Design review of the part built by this model. Coordinates are the model's own, in mm. Face numbers are marked on the shaded views. A direction names the side the tool comes from. Give positions to 0.01 mm unless a question says otherwise; leave off trailing zeros. Loops run counter-clockwise (first coordinate to the right, second up) from the corner with the lowest first, then second, coordinate; pieces in that order, holes last. Notation, with made-up numbers: (-18, 12) -> (8, 12) arc R11 cw to (8, 18) -> close; hole circle Ø4 at (13.25, 39.25). An arc over 180 degrees is marked (long way). Use a Markdown table: item, result. Add a question column.
1. Add section C-C (y = 15.5). State the section outline as (x, z) points.
2. To check wall thickness, follow line 1 (Y direction, x = 6, z = 19.75); line 2 (X direction, y = 8, z = 7.5); line 3 (X direction, y = 17, z = 27). State the ranges of each line that lie inside material, in increasing order.
3. Add section D-D (y = 27.5). State the section outline as (x, z) points.
4. Add section A-A (z = 12). State the section outline as (x, y) points.
5. For the marked faces 5 and 6, list the 3-axis set-ups (+Z, -Z, +X, -X, +Y, -Y) from which the entire face can be reached by the end or side of a thin tool; tool diameter is ignored.
6. For pin 1 Ø12 at (x, y) = (27.5, 25.5) entering from +Z; pin 2 Ø1.6 at (x, y) = (6.5, 27) entering from +Z; pin 3 Ø1.6 at (x, y) = (84, 4.5) entering from +Z; pin 4 Ø4.5 at (x, y) = (13, 16.5) entering from +Z, all flat-tipped, find the tip position at first contact; note any pin that passes through.
7. Draft analysis for pull direction Y (two halves, no side actions). For the marked faces 1, 2, 3 and 4, state which applies: pulls with the +Y half, pulls with the -Y half, needs draft (parallel to the pull), parting line crosses it, or undercut.
8. Add section B-B (x = 84). State the section outline as (y, z) points.
```python
from build123d import *

# Parameters (mm, degrees)
BOX_W           = 90
BOX_H           = 32
BOX_DEPTH       = 35
SKETCH_W        = 82
SKETCH_H        = 27
POCKET_DEPTH    = 30
SKETCH001_W     = 15
SKETCH001_H     = 27
PAD_DEPTH       = 20
SKETCH002_W     = 4
SKETCH002_H     = 4
PAD001_DEPTH    = 4
SKETCH003_W     = 2
SKETCH003_H     = 5
POCKET001_DEPTH = 6
SKETCH004_W     = 4.5
SKETCH004_H     = 2
POCKET002_DEPTH = 13
SKETCH005_W     = 5.5
SKETCH005_H     = 4.5
POCKET003_DEPTH = 2.5
FILLET_R        = 1
SKETCH006_R     = 1
POCKET004_DEPTH = 12
FILLET001_R     = 2


with BuildPart() as part:
    # Box → Box (new body)
    with BuildSketch(Plane.XY):
        with Locations((45, 16)):
            Rectangle(BOX_W, BOX_H)
    extrude(amount=BOX_DEPTH)

    # Sketch (on Face6 of BaseFeature) → Pocket (cut)
    with BuildSketch(Plane.XY.offset(35)):
        with Locations((45, 16)):
            Rectangle(SKETCH_W, SKETCH_H)
    extrude(amount=-POCKET_DEPTH, mode=Mode.SUBTRACT)

    # Sketch001 (on Face11 of Pocket) → Pad (join)
    with BuildSketch(Plane.XY.offset(5)):
        with Locations((11.5, 16)):
            Rectangle(SKETCH001_W, SKETCH001_H)
        with Locations((78.5, 16)):
            Rectangle(SKETCH001_W, SKETCH001_H)
    extrude(amount=PAD_DEPTH)

    # Sketch002 (on Face11 of Pad) → Pad001 (join)
    with BuildSketch(Plane.XY.offset(25)):
        with Locations((6, 27.5)):
            Rectangle(SKETCH002_W, SKETCH002_H)
        with Locations((6, 4.5)):
            Rectangle(SKETCH002_W, SKETCH002_H)
        with Locations((84, 27.5)):
            Rectangle(SKETCH002_W, SKETCH002_H)
        with Locations((84, 4.5)):
            Rectangle(SKETCH002_W, SKETCH002_H)
    extrude(amount=PAD001_DEPTH)

    # Sketch003 (on Face20 of Pad001) → Pocket001 (cut)
    with BuildSketch(Plane.XY.offset(25)):
        with Locations((76.5, 16)):
            Rectangle(SKETCH003_W, SKETCH003_H)
    extrude(amount=-POCKET001_DEPTH, mode=Mode.SUBTRACT)

    # Sketch004 (on Face6 of Pocket001) → Pocket002 (cut)
    with BuildSketch(Plane.YZ.offset(90)):
        with Locations((16, 20)):
            Rectangle(SKETCH004_W, SKETCH004_H)
    extrude(amount=-POCKET002_DEPTH, mode=Mode.SUBTRACT)

    # Sketch005 (on Face6 of Pocket002) → Pocket003 (cut)
    with BuildSketch(Plane.YZ.offset(90)):
        with Locations((16, 20)):
            Rectangle(SKETCH005_W, SKETCH005_H)
    extrude(amount=-POCKET003_DEPTH, mode=Mode.SUBTRACT)

    # Fillet
    fillet_edges = [part.edges().sort_by_distance(p)[0] for p in [
        (88.75, 13.25, 22.25),
        (88.75, 18.75, 22.25),
        (88.75, 13.25, 17.75),
        (88.75, 18.75, 17.75),
    ]]
    fillet(fillet_edges, radius=FILLET_R)

    # Sketch006 (on Face38 of Fillet) → Pocket004 (cut)
    with BuildSketch(Plane.XY.offset(29)):
        with Locations((84, 27.5)):
            Circle(SKETCH006_R)
        with Locations((84, 4.5)):
            Circle(SKETCH006_R)
        with Locations((6, 27.5)):
            Circle(SKETCH006_R)
        with Locations((6, 4.5)):
            Circle(SKETCH006_R)
    extrude(amount=-POCKET004_DEPTH, mode=Mode.SUBTRACT)

    # Fillet001
    fillet001_edges = [part.edges().sort_by_distance(p)[0] for p in [
        (0, 0, 17.5),
        (90, 0, 17.5),
        (90, 32, 17.5),
        (0, 32, 17.5),
    ]]
    fillet(fillet001_edges, radius=FILLET001_R)


solid = part.part
```
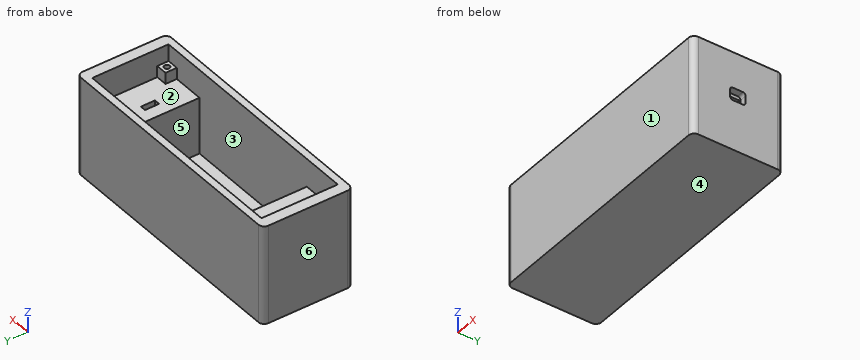
Taken from the geometry:
| question | item | result |
|---|---|---|
| 1 | outline | (0, 0) -> (90, 0) -> (90, 17.75) -> (87.5, 17.75) -> (87.5, 19) -> (75.5, 19) -> (75.5, 25) -> (71, 25) -> (71, 5) -> (19, 5) -> (19, 25) -> (4, 25) -> (4, 35) -> (0, 35) -> close; (77.5, 21) -> (87.5, 21) -> (87.5, 22.25) -> (90, 22.25) -> (90, 35) -> (86, 35) -> (86, 25) -> (77.5, 25) -> close |
| 2 | line 1 | y = 0 to 3.5, 5.5 to 26.5, 28.5 to 32 |
| 2 | line 2 | x = 0 to 19, 71 to 90 |
| 2 | line 3 | x = 0 to 4, 86 to 90 |
| 3 | outline | (0, 0) -> (90, 0) -> (90, 35) -> (86, 35) -> (86, 29) -> (85, 29) -> (85, 17) -> (83, 17) -> (83, 29) -> (82, 29) -> (82, 25) -> (71, 25) -> (71, 5) -> (19, 5) -> (19, 25) -> (8, 25) -> (8, 29) -> (7, 29) -> (7, 17) -> (5, 17) -> (5, 29) -> (4, 29) -> (4, 35) -> (0, 35) -> close |
| 4 | outline | (0, 2) arc R2 ccw to (2, 0) -> (88, 0) arc R2 ccw to (90, 2) -> (90, 30) arc R2 ccw to (88, 32) -> (2, 32) arc R2 ccw to (0, 30) -> close; hole (19, 2.5) -> (71, 2.5) -> (71, 29.5) -> (19, 29.5) -> close |
| 5 | face 5 | +Z |
| 5 | face 6 | +Z, -Z, -X, +Y, -Y |
| 6 | pin 1 | stops at z = 35 |
| 6 | pin 2 | stops at z = 29 |
| 6 | pin 3 | stops at z = 17 |
| 6 | pin 4 | stops at z = 25 |
| 7 | face 1 | pulls with the -Y half |
| 7 | face 2 | undercut |
| 7 | face 3 | undercut |
| 7 | face 4 | needs draft |
| 8 | outline | (0, 0) -> (32, 0) -> (32, 35) -> (29.5, 35) -> (29.5, 29) -> (28.5, 29) -> (28.5, 17) -> (26.5, 17) -> (26.5, 29) -> (25.5, 29) -> (25.5, 25) -> (6.5, 25) -> (6.5, 29) -> (5.5, 29) -> (5.5, 17) -> (3.5, 17) -> (3.5, 29) -> (2.5, 29) -> (2.5, 35) -> (0, 35) -> close; hole (13.75, 19) -> (18.25, 19) -> (18.25, 21) -> (13.75, 21) -> close |
